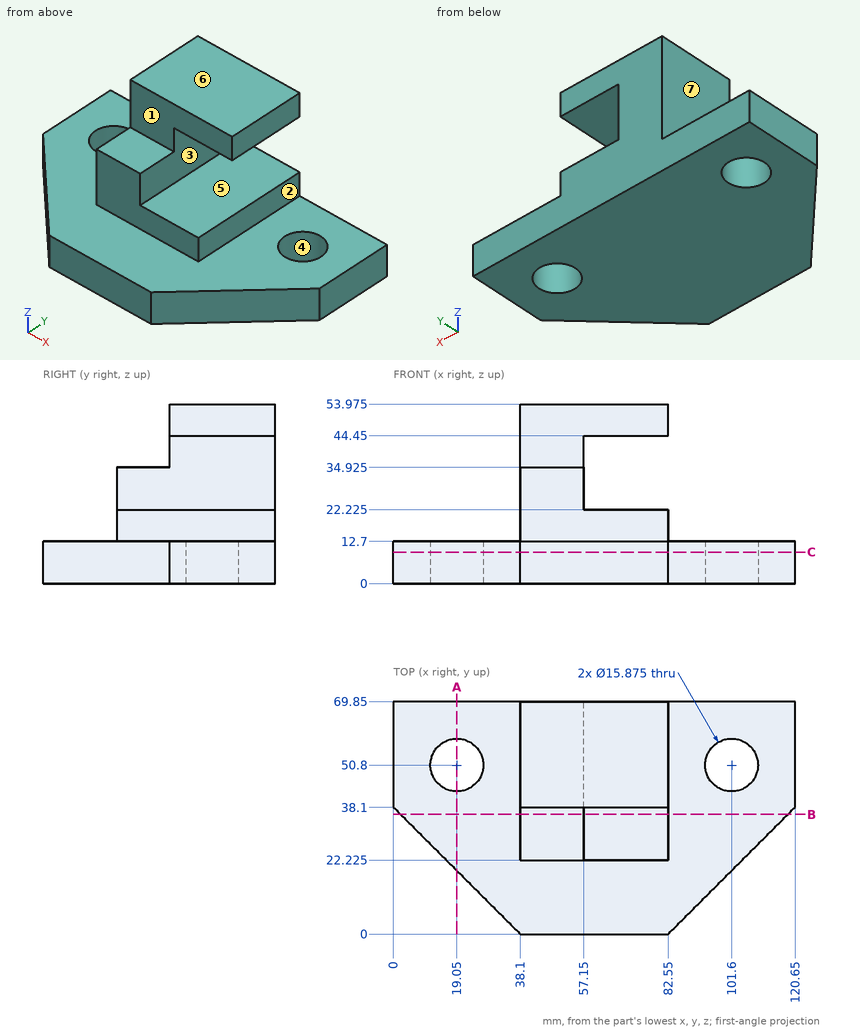
Geometry check sheet. Reference: drawing and pictorial views, mm from the part's lowest x, y, z. A direction names the side the tool comes from. Give positions to 0.01 mm unless a question says otherwise; leave off trailing zeros. Order: outer loops, then holes, each group sorted by start corner. A loop starts at its lowest first (then second) coordinate and runs counter-clockwise, first axis right, second up. Notation, with made-up numbers: M 7.5,-8 L 11.5,-8 A19 cw 11.5,24 Z; hole C -20.75,79 d5. An arc over 180 degrees is marked long. Use one line per item in the form item = value. Start each with the question number.
Q1. Go/stop test with flat-tipped pins: pin 1 Ø17.5 at (x, y) = (45, 27) entering from +Z (3 decimals); pin 2 Ø20.5 at (x, y) = (19.05, 50.8) entering from +Z; pin 3 Ø18 at (x, z) = (67, 23) entering from -Y (3 decimals); pin 4 Ø9.5 at (x, y) = (101.6, 50.8) entering from -Z. Record where each tip stops, or that it passes through.
Q2. Access from +Z, -Z, +X, -X, +Y, -Y to the whole of each face (thin tool, end or side, straight path). Record for the marked faces 1, 2, 3 and 4.
Q3. Section check A-A (x = 19.05). Enter the section's corners in (y, z), then the cut area to 3 significant figures.
Q4. Scan lines: line 1 along Z through (x, y) = (58.5, 46.5) (3 decimals); line 2 along X through (y, z) = (41, 15.5); line 3 along X through (y, z) = (50, 9). Record each from-to range of solid material in increasing order. Write a range as [from, to].
Q5. Mould release check, pull along Z, two halves, no side actions. Record for the marked faces 5, 6 and 7: +Z half, -Z half, draft (parallel to the pull), parting line (faces both ways), or undercut.
Q6. Section check B-B (y = 36). Enter the section's corners in (x, z) (3 decimals), then the cut area to 3 significant figures.
Q7. Section check C-C (z = 9.5). Count the separate pieces of the cut face and the enclosed holes in it, then the cut area to 3 significant figures.
Evaluation:
q1.pin_1 = 34.925
q1.pin_2 = 12.7
q1.pin_3 = 22.225
q1.pin_4 = through
q2.face_1 = +Z, +X, -X, -Y
q2.face_2 = +Z, +X, +Y, -Y
q2.face_3 = +X, +Y, -Y
q2.face_4 = +Z, -Z
q3.outline = M 19.05,0 L 42.86,0 L 42.86,12.7 L 19.05,12.7 Z; M 58.74,0 L 69.85,0 L 69.85,12.7 L 58.74,12.7 Z
q3.area = 444 mm2
q4.line_1 = [0, 22.225], [44.45, 53.975]
q4.line_2 = [38.1, 82.55]
q4.line_3 = [0, 11.15], [26.95, 93.7], [109.5, 120.65]
q5.face_5 = undercut
q5.face_6 = +Z half
q5.face_7 = draft
q6.outline = M 2.1,0 L 118.55,0 L 118.55,12.7 L 82.55,12.7 L 82.55,22.225 L 57.15,22.225 L 57.15,34.925 L 38.1,34.925 L 38.1,12.7 L 2.1,12.7 Z
q6.area = 2,140 mm2
q7.separate_pieces = 1
q7.enclosed_holes = 2
q7.area = 6,580 mm2
